Could you check a few things on this model? Use its own coordinates, in mm. Face numbers are marked on the shaded views. A direction names the side the tool comes from. Give positions to 0.01 mm unless a question says otherwise; leave off trailing zeros. Loops run counter-clockwise (first coordinate to the right, second up) from the corner with the lowest first, then second, coordinate; pieces in that order, holes last. Notation, with made-up numbers: M -34,3 L 7,3 A13 ccw 7,27 Z; hole C 30,-31 d8. An arc over 180 degrees is marked long. Use a Markdown table: item, result. Add a question column.
1) Suppose I cut it at B-B on x = -136.5. List the corners of the cut face in (y, z) for me.
2) Will these pins go through, and if not, where does the flat tip stop? pin 1 Ø5 at (x, z) = (-9.9, 0) entering from +Y; pin 2 Ø12 at (x, y) = (-81.5, 9) entering from +Z; pin 3 Ø12 at (x, z) = (-67, 10.5) entering from +Y.
3) Suppose I cut it at C-C on x = -23. List the corners of the cut face in (y, z) for me.
4) Which directions (+Z, -Z, +X, -X, +Y, -Y) give clear straight access to the entire face, cutting with the end or side of a thin tool? Please do the marked faces 1 and 2.
5) If I drill on line 1 along X through (y, z) = (-7, -12); line 2 along Z through (x, y) = (-53, -7); line 3 along Z through (x, y) = (-9.9, 17), over which ranges is the centre line in solid material (lowest first)? Write a range as [from, to].
```python
from build123d import *

# Parameters (mm, degrees)
F2_SIZE   = 1
F3_SIZE   = 2.24999
F17_D     = 6
F17_DEPTH = 8
F17_TIP   = 1.8025818571
F18_D     = 6
F18_DEPTH = 8
F18_TIP   = 1.8025818571
F19_D     = 6
F19_DEPTH = 8
F19_TIP   = 1.8025818571
F20_D     = 6
F20_DEPTH = 8
F20_TIP   = 1.8025818571
F21_D     = 6
F21_DEPTH = 8
F21_TIP   = 1.8025818571
F22_D     = 6
F22_DEPTH = 8
F22_TIP   = 1.8025818571


# Not quite as in the source:
# - a fillet or chamfer is up to 0.001 mm smaller than in the source, because OpenCascade refuses the exact size


with BuildPart() as f1:
    # F0 (on Top) → F1 (revolve)
    with BuildSketch(Plane.XY):
        Polygon((-160, 0), (0, 0), (0, 19.95), (-19.8, 19.95), (-19.8, 12.6), (-35, 12.6), (-35, 8), (-142.7, 8), (-142.7, 5.75), (-148.2, 5.75), (-148.2, 3.85), (-153.2, 3.85), (-154.5, 5.75), (-160, 5.75), align=None)
    revolve(axis=Axis((-80, 0, 0), (1, 0, 0)))

    # F2
    f2_edges = [f1.edges().sort_by_distance(p)[0] for p in [
        (-160, -5.75, 0),
        (0, -19.95, 0),
        (-35, -12.6, 0),
        (-19.8, -19.95, 0),
    ]]
    chamfer(f2_edges, length=F2_SIZE)

    # F3 (size 2.25 in the source; OpenCascade refuses exactly that, so slightly less here)
    f3_edges = [f1.edges().sort_by_distance(p)[0] for p in [
        (-142.7, -8, 0),
    ]]
    chamfer(f3_edges, length=F3_SIZE)

    # F17
    with Locations(Plane(origin=(0, -19.95, 0), x_dir=(-1, 0, 0), z_dir=(0, -1, 0))):
        with Locations((9.9, 0)):
            Hole(F17_D / 2, depth=F17_DEPTH)
            with Locations((0, 0, -(F17_DEPTH + F17_TIP / 2))):  # 118° drill point
                Cone(0, F17_D / 2, F17_TIP, mode=Mode.SUBTRACT)

    # F18
    with Locations(Plane(origin=(0, -9.975, 17.2772068055), x_dir=(1, 0, 0), z_dir=(0, -0.5, 0.8660254038))):
        with Locations((-9.9, 0)):
            Hole(F18_D / 2, depth=F18_DEPTH)
            with Locations((0, 0, -(F18_DEPTH + F18_TIP / 2))):  # 118° drill point
                Cone(0, F18_D / 2, F18_TIP, mode=Mode.SUBTRACT)

    # F19
    with Locations(Plane(origin=(0, 9.975, 17.2772068055), x_dir=(1, 0, 0), z_dir=(0, 0.5, 0.8660254038))):
        with Locations((-9.9, 0)):
            Hole(F19_D / 2, depth=F19_DEPTH)
            with Locations((0, 0, -(F19_DEPTH + F19_TIP / 2))):  # 118° drill point
                Cone(0, F19_D / 2, F19_TIP, mode=Mode.SUBTRACT)

    # F20
    with Locations(Plane(origin=(0, 19.95, 0), x_dir=(-1, 0, 0), z_dir=(0, 1, 0))):
        with Locations((9.9, 0)):
            Hole(F20_D / 2, depth=F20_DEPTH)
            with Locations((0, 0, -(F20_DEPTH + F20_TIP / 2))):  # 118° drill point
                Cone(0, F20_D / 2, F20_TIP, mode=Mode.SUBTRACT)

    # F21
    with Locations(Plane(origin=(0, 9.975, -17.2772068055), x_dir=(1, 0, 0), z_dir=(0, 0.5, -0.8660254038))):
        with Locations((-9.9, 0)):
            Hole(F21_D / 2, depth=F21_DEPTH)
            with Locations((0, 0, -(F21_DEPTH + F21_TIP / 2))):  # 118° drill point
                Cone(0, F21_D / 2, F21_TIP, mode=Mode.SUBTRACT)

    # F22
    with Locations(Plane(origin=(0, -9.975, -17.2772068055), x_dir=(1, 0, 0), z_dir=(0, -0.5, -0.8660254038))):
        with Locations((-9.9, 0)):
            Hole(F22_D / 2, depth=F22_DEPTH)
            with Locations((0, 0, -(F22_DEPTH + F22_TIP / 2))):  # 118° drill point
                Cone(0, F22_D / 2, F22_TIP, mode=Mode.SUBTRACT)


solid = f1.part
```
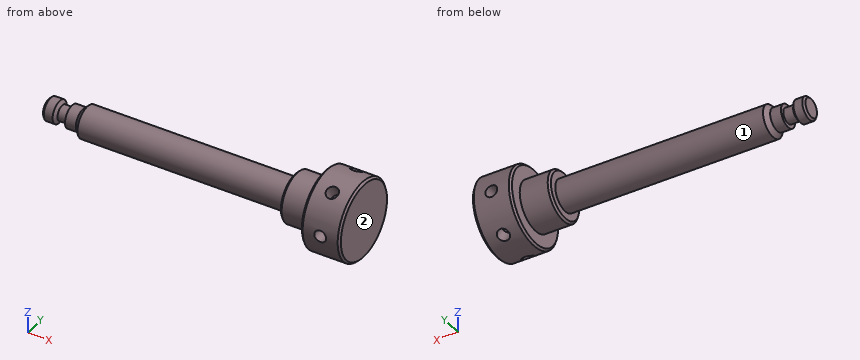
Answer block:
| question | item | result |
|---|---|---|
| 1 | outline | C 0,0 d16 |
| 2 | pin 1 | stops at y = 11.65 |
| 2 | pin 2 | stops at z = 7.42 |
| 2 | pin 3 | stops at y = 6.61 |
| 3 | outline | C 0,0 d25.2 |
| 4 | face 1 | -X |
| 4 | face 2 | +Z, -Z, +X, +Y, -Y |
| 5 | line 1 | x = [-19.8, -12.9], [-6.9, 0] |
| 5 | line 2 | z = [-3.87, 3.87] |
| 5 | line 3 | z = [-10.44, -3], [3, 10.44] |
